Source: CAD feature listing. Evaluate the final solid. Frame: model axes, mm. Face numbers are marked on the shaded views. Coordinates: 2 decimals unless noted, no trailing zeros. Loops run counter-clockwise (first coordinate to the right, second up) from the corner with the lowest first, then second, coordinate; pieces in that order, holes last.
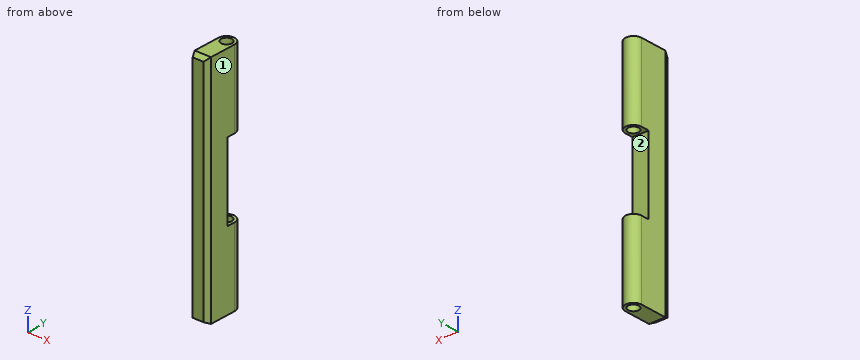
from build123d import *

# Parameters (mm, degrees)
SKETCH1_R               = 1
BOSS_EXTRUDE1_DEPTH     = 42
CUT_EXTRUDE1_DEPTH      = 43.253492101
CUT_EXTRUDE1_DEPTH_BACK = 43.253492101
SKETCH2_W               = 14
SKETCH2_H               = 3
CHAMFER1_SIZE           = 0.5
CHAMFER1_SIZE2          = 1


with BuildPart() as part:
    # Sketch1 → Boss-Extrude1 (new body)
    with BuildSketch(Plane.XY):
        with BuildLine():
            Line((-1.5, 2.871223481), (-1.5, -3.128776519))
            Line((-1.5, -3.128776519), (1.5, -3.128776519))
            Line((1.5, -3.128776519), (1.5, 2.871223481))
            ThreePointArc((1.5, 2.871223481), (0, 4.371223481), (-1.5, 2.871223481))
        make_face()
        with Locations(Location((0, 2.871223481, 0), (0, 0, 180))):
            Circle(SKETCH1_R, mode=Mode.SUBTRACT)
    extrude(amount=BOSS_EXTRUDE1_DEPTH)

    # Sketch2 → Cut-Extrude1 (cut, two sides: drawn at the far end of the back side and taken through both)
    with BuildSketch(Plane(origin=(0, 0, 0), x_dir=(0, 0, -1), z_dir=(1, 0, 0)).offset(-CUT_EXTRUDE1_DEPTH_BACK)):
        with Locations((-21, 2.871223481)):
            Rectangle(SKETCH2_W, SKETCH2_H)
    extrude(amount=CUT_EXTRUDE1_DEPTH + CUT_EXTRUDE1_DEPTH_BACK, mode=Mode.SUBTRACT)

    # Chamfer1
    chamfer1_edges = [part.edges().sort_by_distance(p)[0] for p in [
        (0, -3.128776519, 42),
        (0, -3.128776519, 0),
        (1.5, -3.128776519, 21),
        (-1.5, -3.128776519, 21),
    ]]
    chamfer1_side = [part.faces().sort_by_distance(p)[0] for p in [
        (0, -3.128776519, 21),
    ]]
    chamfer(chamfer1_edges, length=CHAMFER1_SIZE, length2=CHAMFER1_SIZE2, reference=chamfer1_side[0])


solid = part.part
Q1. Section B-B, the plane z = 4.5. Return the cut outline in (x, y).
Q2. Section C-C, the plane z = 23.5. Return the cut outline in (x, y).
Q3. Section A-A, the plane x = 0. Return the cut outline in (y, z).
Q4. Draft query along Z for the marked faces 1 and 2. Return one class per face: +Z half, -Z half, draft (parallel to the pull), parting line (faces both ways), or undercut.
Q5. Contact query for flat-ended pins moving along their axis: pin 1 Ø1.5 at (x, z) = (-1, 5) entering from +Y; pin 2 Ø1.5 at (x, z) = (-0.5, 21.5) entering from +Y. Output: stop coordinate, or through.
Q6. Line query: line 1 along X through (y, z) = (3, 39); line 2 along Y through (x, z) = (0, 7.5); line 3 along Z through (x, y) = (-0.8, 1.5). Output: solid intervals per line, ascending.
Derived:
1. outline: (-1.5, -2.13) - (-1, -3.13) - (1, -3.13) - (1.5, -2.13) - (1.5, 2.87) arc R1.5 ccw to (-1.5, 2.87) - close; hole circle Ø2 at (0, 2.87)
2. outline: (-1.5, -2.13) - (-1, -3.13) - (1, -3.13) - (1.5, -2.13) - (1.5, 1.37) - (-1.5, 1.37) - close
3. outline: (-3.13, 0.5) - (-2.13, 0) - (1.87, 0) - (1.87, 14) - (1.37, 14) - (1.37, 28) - (1.87, 28) - (1.87, 42) - (-2.13, 42) - (-3.13, 41.5) - close; (3.87, 0) - (4.37, 0) - (4.37, 14) - (3.87, 14) - close; (3.87, 28) - (4.37, 28) - (4.37, 42) - (3.87, 42) - close
4. face 1: draft
4. face 2: undercut
5. pin 1: stops at y = 4.35
5. pin 2: stops at y = 1.37
6. line 1: x = -1.49 to -0.99, 0.99 to 1.49
6. line 2: y = -3.13 to 1.87, 3.87 to 4.37
6. line 3: z = 0 to 14, 28 to 42
